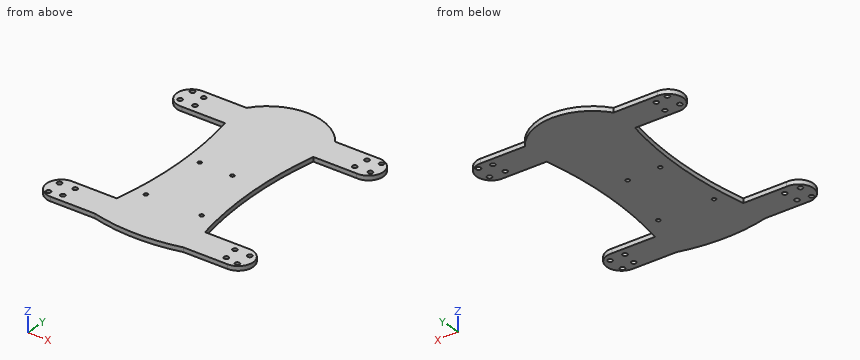
```python
from build123d import *

# Parameters (mm, degrees)
F0_R     = 2
F0_R_2   = 1.651
F1_DEPTH = 3.81


with BuildPart() as f1:
    # F0 (on Top) → F1 (new body)
    with BuildSketch(Plane.XY):
        with BuildLine():
            ThreePointArc((37.946905, 88.097033), (-0.153095, 107.714284), (-38.253095, 88.097033))
            Line((-38.253095, 88.097033), (-37.946905, 88.097033))
            Line((-37.946905, 88.097033), (37.946905, 88.097033))
        make_face()
        Polygon((-37.946905, 88.097033), (-38.253095, 88.097033), (-37.946905, 62.742965), (37.946905, 62.742965), (37.946905, 88.097033), align=None)
        with BuildLine():
            Line((-37.946905, 62.742965), (-38.253095, 88.097033))
            Line((-38.253095, 88.097033), (-76.046905, 88.097033))
            ThreePointArc((-76.046905, 88.097033), (-88.735417, 74.856974), (-74.967762, 62.742965))
            Line((-74.967762, 62.742965), (-37.946905, 62.742965))
        make_face()
        with Locations((-81.778049, 69.815444)):
            Circle(F0_R, mode=Mode.SUBTRACT)
        with Locations((-68.661721, 69.381662)):
            Circle(F0_R, mode=Mode.SUBTRACT)
        with Locations((-70.195213, 81.486084)):
            Circle(F0_R, mode=Mode.SUBTRACT)
        with Locations((-81.191262, 83.413343)):
            Circle(F0_R, mode=Mode.SUBTRACT)
        with BuildLine():
            Line((76.046905, 88.097033), (37.946905, 88.097033))
            Line((37.946905, 88.097033), (37.946905, 62.742965))
            Line((37.946905, 62.742965), (74.967762, 62.742965))
            ThreePointArc((74.967762, 62.742965), (88.735417, 74.856974), (76.046905, 88.097033))
        make_face()
        with Locations((68.661721, 69.381662)):
            Circle(F0_R, mode=Mode.SUBTRACT)
        with Locations((81.778049, 69.815444)):
            Circle(F0_R, mode=Mode.SUBTRACT)
        with Locations((70.195213, 81.486084)):
            Circle(F0_R, mode=Mode.SUBTRACT)
        with Locations((81.191262, 83.413343)):
            Circle(F0_R, mode=Mode.SUBTRACT)
        with BuildLine():
            Line((-37.946905, -88.097033), (-37.946905, -62.742965))
            Line((-37.946905, -62.742965), (-74.967762, -62.742965))
            ThreePointArc((-74.967762, -62.742965), (-88.735417, -74.856974), (-76.046905, -88.097033))
            Line((-76.046905, -88.097033), (-37.946905, -88.097033))
        make_face()
        with Locations((-81.191262, -83.413343)):
            Circle(F0_R, mode=Mode.SUBTRACT)
        with Locations((-70.195213, -81.486084)):
            Circle(F0_R, mode=Mode.SUBTRACT)
        with Locations((-81.778049, -69.815444)):
            Circle(F0_R, mode=Mode.SUBTRACT)
        with Locations((-68.661721, -69.381662)):
            Circle(F0_R, mode=Mode.SUBTRACT)
        with BuildLine():
            Line((74.967762, -62.742965), (37.946905, -62.742965))
            Line((37.946905, -62.742965), (38.253095, -88.097033))
            Line((38.253095, -88.097033), (76.046905, -88.097033))
            ThreePointArc((76.046905, -88.097033), (88.735417, -74.856974), (74.967762, -62.742965))
        make_face()
        with Locations((70.195213, -81.486084)):
            Circle(F0_R, mode=Mode.SUBTRACT)
        with Locations((81.191262, -83.413343)):
            Circle(F0_R, mode=Mode.SUBTRACT)
        with Locations((68.661721, -69.381662)):
            Circle(F0_R, mode=Mode.SUBTRACT)
        with Locations((81.778049, -69.815444)):
            Circle(F0_R, mode=Mode.SUBTRACT)
        Polygon((37.946905, -62.742965), (-37.946905, -62.742965), (-37.946905, -88.097033), (37.946905, -88.097033), (38.253095, -88.097033), align=None)
        with BuildLine():
            Line((37.946905, -88.097033), (-37.946905, -88.097033))
            ThreePointArc((-37.946905, -88.097033), (0.153095, -92.851298), (38.253095, -88.097033))
            Line((38.253095, -88.097033), (37.946905, -88.097033))
        make_face()
        with BuildLine():
            Line((37.946905, 62.742965), (-37.946905, 62.742965))
            ThreePointArc((-37.946905, 62.742965), (-31.75, 0), (-37.946905, -62.742965))
            Line((-37.946905, -62.742965), (37.946905, -62.742965))
            ThreePointArc((37.946905, -62.742965), (31.75, 0), (37.946905, 62.742965))
        make_face()
        with Locations((-24.873505, -46.499295)):
            Circle(F0_R_2, mode=Mode.SUBTRACT)
        with Locations((22.802295, -46.141523)):
            Circle(F0_R_2, mode=Mode.SUBTRACT)
        with Locations((-20.59705, 9.981038)):
            Circle(F0_R_2, mode=Mode.SUBTRACT)
        with Locations((7.97795, 9.401235)):
            Circle(F0_R_2, mode=Mode.SUBTRACT)
    extrude(amount=F1_DEPTH)


solid = f1.part
```
CAD build for the part. Positions are in the model's coordinates, mm. Round coordinates to 2 decimals unless told otherwise and drop trailing zeros. Loops run counter-clockwise (first coordinate to the right, second up) from the corner with the lowest first, then second, coordinate; pieces in that order, holes last. Notation, with made-up numbers: M 82.25,87 L 102.25,87 A20 cw 102.25,112 Z; hole C -24.75,22 d11. An arc over 180 degrees is marked long. Return JSON: item names as keys, results as strings. Group by question number.
(1) Saw through at C-C, the plane z = 0.6. Give the number of separate pieces and of enclosed holes in the cut face, and give its area (3 significant figures).
(2) Saw through at A-A, the plane x = 48. List the corners of the cut face in (y, z).
(3) Wall check: probe 1 along Y at (x, z) = (65, 2.15); probe 2 along X at (y, z) = (-83, 1.4); probe 3 along Y at (x, z) = (-81, 1.6). Give the ranges that are in metal, low to high. Write a range as [from, to].
(4) Saw through at D-D, the plane x = 29. List the corners of the cut face in (y, z).
(5) Saw through at B-B, the plane y = 34. List the corners of the cut face in (x, z), and give its area (3 significant figures).
(6) Drop flat-ended pins along their axis: P1, Ø1.9, axis at x = 61.5, z = 2.5, coming from the -Y side; P2, Ø2, axis at y = -50.5, z = 1, coming from the -X side. Give the stop position or say it passes through.
Answer list:
{
 "1": {"separate pieces": "1", "enclosed holes": "20", "area": "18,300 mm2"},
 "2": {"outline": "M -88.1,0 L -62.74,0 L -62.74,3.81 L -88.1,3.81 Z; M 62.74,0 L 88.1,0 L 88.1,3.81 L 62.74,3.81 Z"},
 "3": {"probe 1": "[-88.1, -62.74], [62.74, 88.1]", "probe 2": "[-86.22, -83.15], [-79.23, -71.5], [-68.89, 68.89], [71.5, 79.23], [83.15, 86.22]", "probe 3": "[-87.09, -85.4], [-81.42, -71.66], [-67.97, -63.7], [63.7, 67.97], [71.66, 81.42], [85.4, 87.09]"},
 "4": {"outline": "M -90.14,0 L 97.53,0 L 97.53,3.81 L -90.14,3.81 Z"},
 "5": {"outline": "M -33.56,0 L 33.56,0 L 33.56,3.81 L -33.56,3.81 Z", "area": "256 mm2"},
 "6": {"P1": "y = -88.1", "P2": "x = -35.91"}
}
